```python
from build123d import *

# Parameters (mm, degrees)
SKETCH1_W           = 118
SKETCH1_H           = 10
BOSS_EXTRUDE1_DEPTH = 116
BOSS_EXTRUDE2_DEPTH = 46
SKETCH3_R           = 14
CUT_EXTRUDE1_DEPTH  = 195.117634996
SKETCH4_R           = 29.5
SKETCH4_R_2         = 25.5
BOSS_EXTRUDE3_DEPTH = 67
SKETCH6_W           = 44
SKETCH6_H           = 30
BOSS_EXTRUDE4_DEPTH = 55
CUT_EXTRUDE2_START  = -44
CUT_EXTRUDE2_DEPTH  = 44


with BuildPart() as part:
    # Sketch1 → Boss-Extrude1 (new body)
    with BuildSketch(Plane.XY):
        with Locations((-0.073312219, 5)):
            Rectangle(SKETCH1_W, SKETCH1_H)
    extrude(amount=-BOSS_EXTRUDE1_DEPTH)

    # Sketch2 → Boss-Extrude2 (add)
    with BuildSketch(Plane(origin=(10, 0, 0), x_dir=(0, 0, -1), z_dir=(1, 0, 0))):
        with BuildLine():
            Line((0, 86), (0, 10))
            Line((0, 10), (116, 10))
            Line((116, 10), (116, 86))
            ThreePointArc((116, 86), (58, 144), (0, 86))
        make_face()
    extrude(amount=-BOSS_EXTRUDE2_DEPTH)

    # Sketch3 → Cut-Extrude1 (cut, through all)
    with BuildSketch(Plane.XY):
        with Locations((-13, 24)):
            Circle(SKETCH3_R)
    extrude(amount=-CUT_EXTRUDE1_DEPTH, mode=Mode.SUBTRACT)

    # Sketch4 → Boss-Extrude3 (add)
    with BuildSketch(Plane(origin=(10, 0, 0), x_dir=(0, 0, -1), z_dir=(1, 0, 0))):
        with Locations((58, 86)):
            Circle(SKETCH4_R)
        with Locations((58, 86)):
            Circle(SKETCH4_R_2, mode=Mode.SUBTRACT)
    extrude(amount=BOSS_EXTRUDE3_DEPTH)

    # Sketch6 → Boss-Extrude4 (add)
    with BuildSketch(Plane(origin=(0, 10, 0), x_dir=(1, 0, 0), z_dir=(0, 1, 0))):
        with Locations((32, 57.975103421)):
            Rectangle(SKETCH6_W, SKETCH6_H)
    extrude(amount=BOSS_EXTRUDE4_DEPTH)

    # Sketch7 → Cut-Extrude2 (cut)
    with BuildSketch(Plane(origin=(54, 0, 0), x_dir=(0, 0, -1), z_dir=(1, 0, 0)).offset(CUT_EXTRUDE2_START)):
        with BuildLine():
            Line((43.534523859, 65), (72.465476141, 65))
            ThreePointArc((72.465476141, 65), (58, 60.5), (43.534523859, 65))
        make_face()
    extrude(amount=CUT_EXTRUDE2_DEPTH, mode=Mode.SUBTRACT)


solid = part.part
```
CAD build for the part. Positions are in the model's coordinates, mm. A direction names the side the tool comes from. Coordinates: 2 decimals unless noted, no trailing zeros. Write each loop counter-clockwise with the first axis right and the second up, starting at its lowest first coordinate (ties: lowest second). Pieces come first, ordered by that corner, then holes.
(1) Two-plate mould, pull along Z, no slides. Class faces 6 (the face through (10, 86, -58)), 7 (the face through (-9, 43, 0)), 8 (the face through (43.03, 115.25, -54.16)), 9 (the face through (54, 35, -58)): +Z half, -Z half, draft (parallel to the pull), parting line (faces both ways), or undercut.
(2) Drill centre lines: probe 1 along X at (y, z) = (119, -54.5); probe 2 along Z at (x, y) = (24, 86); probe 3 along X at (y, z) = (9.5, -4.5). Where is each one in solid material? Low to high.
(3) Cut at B-B, the plane y = 24. List the corners of the cut face in (x, z).
(4) Flat gauge pins, fed straight in: pin 1 (3 mm diameter, centred on y = 119.5, z = -92.5, fed in from -X); pin 2 (10 mm diameter, centred on x = 14.5, z = -58.5, fed in from +Y); pin 3 (3 mm diameter, centred on y = 16, z = -28.5, fed in from +X). Where does each tip first touch, or does it go through?
(5) Cut at C-C, the plane z = -58. List the corners of the cut face in (x, y), and give its area (3 significant figures).
(6) Cut at A-A, the plane x = -13. List the corners of the cut face in (y, z), and give its area (3 significant figures).
(7) 3-axis set-ups, long thin cutter, end or side, ignore diameter. For faces 1 (the face through (-48, 10, -57)), 2 (the face through (32, 35, -42.975)), 3 (the face through (58.927, 5, -57)), 4 (the face through (56, 10, -57)), 5 (the face through (32, 35, -72.975)): which of +Z, -Z, +X, -X, +Y, -Y reach the whole face in a straight line?
(8) Cut at D-D, the plane x = 16. List the corners of the cut face in (y, z).
Geometry says:
1. face 6: undercut
1. face 7: +Z half
1. face 8: parting line
1. face 9: draft
2. probe 1: x = -36 to 10
2. probe 2: z = -87.5 to -83.5, -32.5 to -28.5
2. probe 3: x = -59.07 to 58.93
3. outline: (-36, -116) - (-27, -116) - (-27, 0) - (-36, 0) - close; (1, -116) - (10, -116) - (10, -72.98) - (54, -72.98) - (54, -42.98) - (10, -42.98) - (10, 0) - (1, 0) - close
4. pin 1: stops at x = -36
4. pin 2: stops at y = 144
4. pin 3: stops at x = 10
5. outline: (-59.07, 0) - (58.93, 0) - (58.93, 10) - (54, 10) - (54, 56.5) - (77, 56.5) - (77, 60.5) - (10, 60.5) - (10, 111.5) - (77, 111.5) - (77, 115.5) - (10, 115.5) - (10, 144) - (-36, 144) - (-36, 10) - (-59.07, 10) - close; hole circle Ø28 at (-13, 24)
5. area: 9,310 mm2
6. outline: (0, -116) - (10, -116) - (10, 0) - (0, 0) - close; (38, -116) - (86, -116) arc R58 ccw to (86, 0) - (38, 0) - close
6. area: 12,000 mm2
7. face 1: +Z, -Z, -X, +Y
7. face 2: +Z, +X
7. face 3: +Z, -Z, +X, -Y
7. face 4: +X
7. face 5: -Z, +X
8. outline: (0, -116) - (10, -116) - (10, -72.98) - (60.58, -72.98) arc R29.5 ccw (long way) to (60.61, -42.98) - (10, -42.98) - (10, 0) - (0, 0) - close; hole circle Ø51 at (86, -58)
